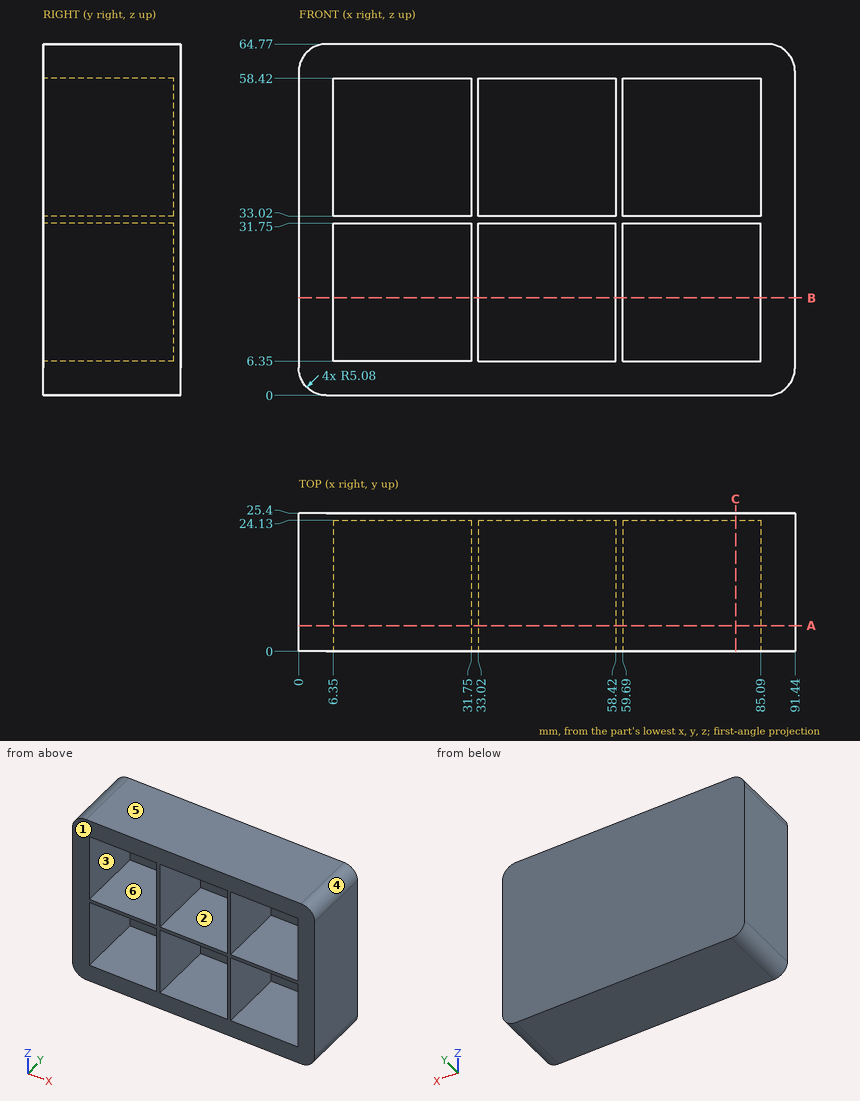
The drawing under review shows one solid part. Ordinate dimensions are in mm from its lowest x, y, z. A direction names the side the tool comes from. Coordinates: 2 decimals unless noted, no trailing zeros. Loops run counter-clockwise (first coordinate to the right, second up) from the corner with the lowest first, then second, coordinate; pieces in that order, holes last. Notation, with made-up numbers: (53.25, 2.5) -> (94.25, 2.5) arc R13 cw to (94.25, 14.5) -> close; hole circle Ø2 at (-35.75, 18). An arc over 180 degrees is marked (long way). Answer as a JSON object with one key per item and string values.
Q1. Tool access review of the marked faces 5 and 6: name each direction out of +Z, -Z, +X, -X, +Y, -Y from which nothing blocks a thin tool from reaching the whole face with its end or side.
Answer block:
{"face 5": "+Z, +X, -X, +Y, -Y", "face 6": "-Y"}
Q2. Take a section at C-C on x = 80.5. Give the boundary of the cut face in (y, z).
Answer block:
{"outline": "(0, 0) -> (25.4, 0) -> (25.4, 64.77) -> (0, 64.77) -> (0, 58.42) -> (24.13, 58.42) -> (24.13, 33.02) -> (0, 33.02) -> (0, 31.75) -> (24.13, 31.75) -> (24.13, 6.35) -> (0, 6.35) -> close"}
Q3. Take a section at B-B on z = 18. Give the boundary of the cut face in (x, y).
Answer block:
{"outline": "(0, 0) -> (6.35, 0) -> (6.35, 24.13) -> (31.75, 24.13) -> (31.75, 0) -> (33.02, 0) -> (33.02, 24.13) -> (58.42, 24.13) -> (58.42, 0) -> (59.69, 0) -> (59.69, 24.13) -> (85.09, 24.13) -> (85.09, 0) -> (91.44, 0) -> (91.44, 25.4) -> (0, 25.4) -> close"}
Q4. The part is to be moulded in two halves that separate along Z. For the marked faces 1, 2, 3 and 4, say which applies: +Z half, -Z half, draft (parallel to the pull), parting line (faces both ways), or undercut.
Answer block:
{"face 1": "draft", "face 2": "undercut", "face 3": "undercut", "face 4": "+Z half"}
Q5. Clearance check with flat-ended pins moving along their axes: pin 1 Ø12 at (x, y) = (29, 12) entering from -Z; pin 2 Ø12.5 at (x, z) = (13.5, 45.5) entering from -Y. State where each tip first meets the part, or that it passes through.
Answer block:
{"pin 1": "stops at z = 0", "pin 2": "stops at y = 24.13"}
Q6. Take a section at A-A on y = 4.75. Give the number of separate pieces and of enclosed holes in the cut face, plus the area to 3 significant figures.
Answer block:
{"separate pieces": "1", "enclosed holes": "6", "area": "2,030 mm^2"}
Q7. To check wall thickness, follow L1, parallel to X at y = 11.75, z = 29.5; L2, parallel to Z at x = 53, y = 7.5; L3, parallel to Y at x = 84, z = 13.5. State the ranges of each line that lie inside material, in increasing order.
Answer block:
{"L1": "x = 0 to 6.35, 31.75 to 33.02, 58.42 to 59.69, 85.09 to 91.44", "L2": "z = 0 to 6.35, 31.75 to 33.02, 58.42 to 64.77", "L3": "y = 24.13 to 25.4"}
